Autodesk Inventor part; units mm, degrees
ref_plane "YZ Plane" through (0, 0, 0) normal (1, 0, 0) x (0, 1, 0)
ref_plane "XZ Plane" through (0, 0, 0) normal (0, 1, 0) x (-1, 0, 0)
ref_plane "XY Plane" through (0, 0, 0) normal (0, 0, 1) x (1, 0, 0)
sketch "Skizze1" plane through (0, 0, 0) normal (0, 0, 1) x (1, 0, 0)
  circle A0 centre (0, 0) radius 11.1 construction
  circle A1 centre (0, 0) radius 25
  circle A2 centre (0, 0) radius 15
  circle A3 centre (-15, -15) radius 1.25
  circle A4 centre (15, 15) radius 1.25
  circle A5 centre (15, -15) radius 1.25
  circle A6 centre (-15, 15) radius 1.25
  point P0 (0, 0)
  dimension "d0" = 30
extrude "Extrusion1" add sketch "Skizze1" along normal blind 9 contours A1 | A3 | A4 | A5 | A6
sketch "Skizze2" plane through (0, 0, 9) normal (0, 0, 1) x (1, 0, 0)
  circle A0 centre (0, 0) radius 15
  circle A1 centre (0, 0) radius 25
  point P0 (0, 0)
extrude "Extrusion2" add sketch "Skizze2" against normal blind 2 contours A0
fillet "Rundung1" radius 5 1 edges at (-25, 0, 9)
sketch "Skizze3" plane through (0, 0, 9) normal (0, 0, 1) x (1, 0, 0)
  line L0 (-15, -15) -> (15, -15)
  line L1 (15, -15) -> (15, 15)
  line L2 (15, 15) -> (-15, 15)
  line L3 (-15, 15) -> (-15, -15)
  line L4 (-15, -15) -> (15, 15) construction
  line L5 (15, -15) -> (-15, 15) construction
  point P0 (0, 0)
  dimension "d6" = 30
hole "Bohrung1" at (-15, 15, 9) at (15, 15, 9) at (15, -15, 9) at (-15, -15, 9) direction (0, 0, -1) diameter 3 end through all counterbore diameter 6 counterbore depth 4
properties part number "Cover_G2" material "ABS-Kunststoff"
Build history of the part. All positions in model axes, mm. A direction names the side the tool comes from. Round coordinates to 2 decimals unless told otherwise and drop trailing zeros. Loops run counter-clockwise (first coordinate to the right, second up) from the corner with the lowest first, then second, coordinate; pieces in that order, holes last.
Item 1: Saw through at B-B (y = 0). List the corners of the cut face in (x, z).
Item 2: Drill centre lines: line 1 along X through (y, z) = (-16, 5.25); line 2 along X through (y, z) = (-17.5, 5.75); line 3 along Z through (x, y) = (-6.5, -12). Where is each one in solid material? Low to high.
Item 3: Two-plate mould, pull along Y, no slides. Class faces 4 (the face through (16.3, 13.7, 5)), 5 (the face through (11, -11, 0)), 6 (the face through (23.846, -7.509, 1.972)): released by +Y, released by -Y, zero draft, split by the parting line, or undercut.
Item 4: Saw through at C-C (z = 8.25). List the corners of the cut face in (x, y).
Item 5: Which spindle directions (+Z, -Z, +X, -X, +Y, -Y) get a long thin tool onto all of the face, cutting with end or side? Do faces 1 (the face through (-14.985, -0.66, 3.451)), 2 (the face through (14.93, -13.5, 2.46)), 3 (the face through (-13.2, -12.6, 7)). Say none if no direction does.
Item 6: Pin check, flat tips, straight feed: P1, Ø4, axis at x = 15, y = -15, coming from the +Z side; P2, Ø5, axis at x = 14.5, y = 13.5, coming from the +Z side; P3, Ø1.5, axis at x = -5.5, z = 1, coming from the +Y side; P4, Ø4, axis at x = 8.5, y = 4.5, coming from the -Z side. Stop position of each tip, or through.
Item 7: Saw through at A-A (z = 3). List the corners of the cut face in (x, y), then the cut area to 3 significant figures.
Worked answers:
1. outline: (-25, 0) - (-15, 0) - (-15, 7) - (15, 7) - (15, 0) - (25, 0) - (25, 4) arc R5 ccw to (20, 9) - (-20, 9) arc R5 ccw to (-25, 4) - close
2. line 1: x = -19 to -17.83, -12.17 to 12.17, 17.83 to 19
2. line 2: x = -17.41 to -16.66, -13.34 to 13.34, 16.66 to 17.41
2. line 3: z = 7 to 9
3. face 4: undercut
3. face 5: zero draft
3. face 6: split by the parting line
4. outline: (-17.81, -13.96) arc R3 cw (long way) to (-13.96, -17.81) arc R22.63 ccw to (13.96, -17.81) arc R3 cw (long way) to (17.81, -13.96) arc R22.63 ccw to (17.81, 13.96) arc R3 cw (long way) to (13.96, 17.81) arc R22.63 ccw to (-13.96, 17.81) arc R3 cw (long way) to (-17.81, 13.96) arc R22.63 ccw to start
5. face 1: -Z
5. face 2: +Z, -Z
5. face 3: +Z
6. P1: stops at z = 5
6. P2: stops at z = 9
6. P3: stops at y = 24.54
6. P4: stops at z = 7
7. outline: circle Ø50 at (0, 0); hole circle Ø3 at (-15, -15); hole circle Ø3 at (-15, 15); hole circle Ø30 at (0, 0); hole circle Ø3 at (15, -15); hole circle Ø3 at (15, 15)
7. area: 1,230 mm2
